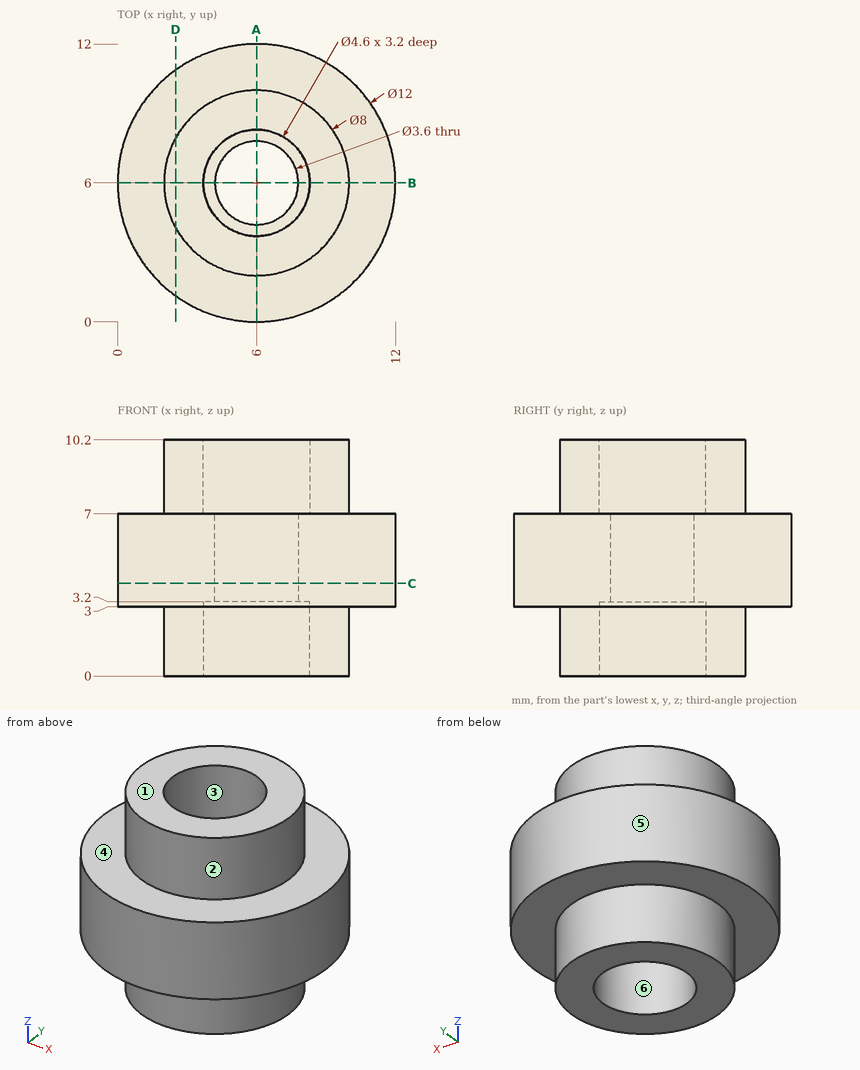
Source: three-view drawing plus pictorial views. Frame: mm from the lowest corner of the part. A direction names the side the tool comes from. Coordinates: 2 decimals unless noted, no trailing zeros. Loops run counter-clockwise (first coordinate to the right, second up) from the corner with the lowest first, then second, coordinate; pieces in that order, holes last. Notation, with made-up numbers: (-1, 41) - (14, 41) arc R24 ccw to (14, 62) - close; hole circle Ø3 at (17, -5). An arc over 180 degrees is marked (long way). Answer in a Markdown table with one row per item. Add a question column.
Item 1: Section query D-D on x = 2.5. Return the cut outline in (y, z), then the cut area to 3 significant figures.
Item 2: Section query C-C on z = 4. Return the cut outline in (x, y), then the cut area to 3 significant figures.
Item 3: Access query for the marked faces 4, 5 and 6. Directions: +Z, -Z, +X, -X, +Y, -Y. A direction counts if a zero-diameter tool reaches every point of the face in a straight line with its end or side. Return the directions, or none.
Item 4: Contact query for flat-ended pins moving along their axis: P1, Ø3, axis at y = 4.5, z = 9, coming from the +X side; P2, Ø3, axis at x = 6, y = 6, coming from the -Z side; P3, Ø1, axis at x = 2.5, z = 8.5, coming from the +Y side; P4, Ø5, axis at x = 9.5, z = 7, coming from the -Y side. Output: stop coordinate, or through.
Item 5: Line query: line 1 along Y through (x, z) = (6, 8); line 2 along Z through (x, y) = (11.5, 8.25); line 3 along Y through (x, z) = (5.5, 7.5) (3 decimals). Output: solid intervals per line, ascending. Write a range as [from, to].
Item 6: Section query A-A on x = 6. Return the cut outline in (y, z), then the cut area to 3 significant figures.
Item 7: Mould query, pull axis Y, two halves, no side actions, for the marked faces 1, 2 and 3. Classes: released by +Y, released by -Y, zero draft, split by the parting line, or undercut.
Recorded:
| question | item | result |
|---|---|---|
| 1 | outline | (1.13, 3) - (4.06, 3) - (4.06, 0) - (7.94, 0) - (7.94, 3) - (10.87, 3) - (10.87, 7) - (7.94, 7) - (7.94, 10.2) - (4.06, 10.2) - (4.06, 7) - (1.13, 7) - close |
| 1 | area | 63.0 mm^2 |
| 2 | outline | circle Ø12 at (6, 6); hole circle Ø3.6 at (6, 6) |
| 2 | area | 103 mm^2 |
| 3 | face 4 | +Z |
| 3 | face 5 | +Z, -Z |
| 3 | face 6 | -Z |
| 4 | P1 | x = 10 |
| 4 | P2 | through |
| 4 | P3 | y = 8.65 |
| 4 | P4 | y = 0.08 |
| 5 | line 1 | [2, 3.7], [8.3, 10] |
| 5 | line 2 | [3, 7] |
| 5 | line 3 | [2.031, 3.755], [8.245, 9.969] |
| 6 | outline | (0, 3) - (2, 3) - (2, 0) - (3.7, 0) - (3.7, 3.2) - (4.2, 3.2) - (4.2, 7) - (3.7, 7) - (3.7, 10.2) - (2, 10.2) - (2, 7) - (0, 7) - close; (7.8, 3.2) - (8.3, 3.2) - (8.3, 0) - (10, 0) - (10, 3) - (12, 3) - (12, 7) - (10, 7) - (10, 10.2) - (8.3, 10.2) - (8.3, 7) - (7.8, 7) - close |
| 6 | area | 54.5 mm^2 |
| 7 | face 1 | zero draft |
| 7 | face 2 | split by the parting line |
| 7 | face 3 | undercut |
